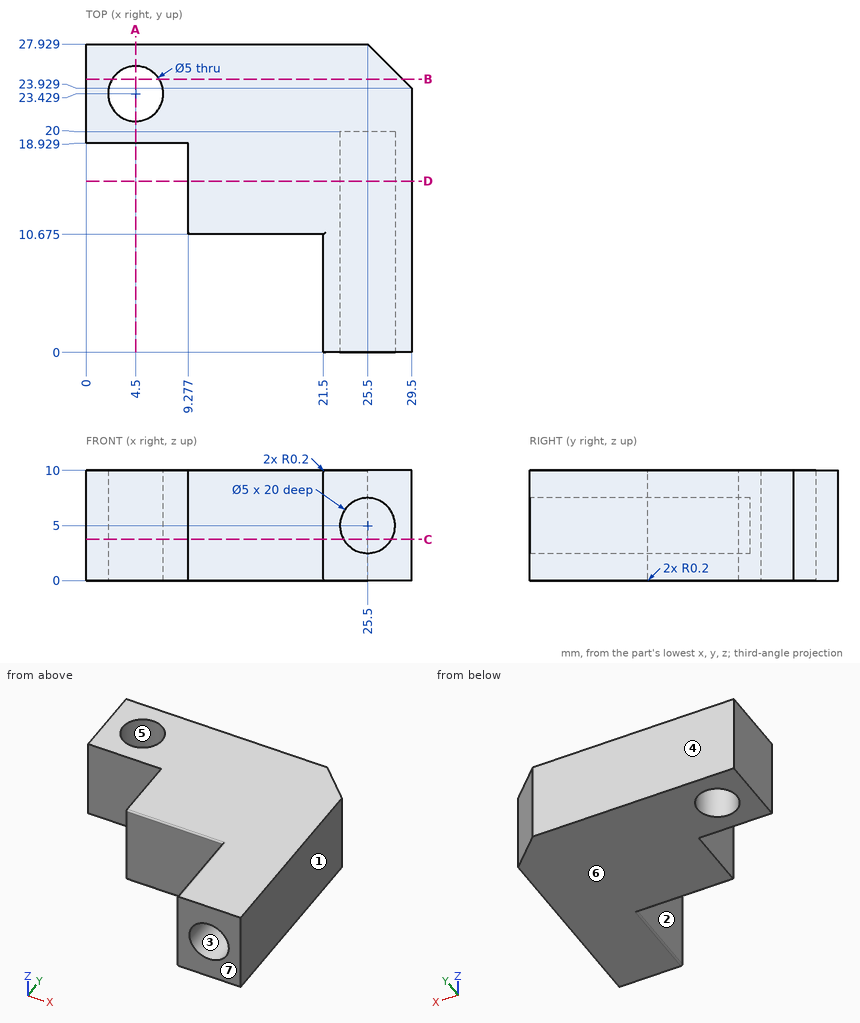
Can you work these out from the drawing? Everything is in mm from the part's minimum corner. A direction names the side the tool comes from. Give positions to 0.01 mm unless a question says otherwise; leave off trailing zeros. Order: outer loops, then holes, each group sorted by start corner. A loop starts at its lowest first (then second) coordinate and runs counter-clockwise, first axis right, second up. Notation, with made-up numbers: M 86.25,20 L 145.25,20 A8 cw 145.25,34 Z; hole C 71.5,11.25 d11. An arc over 180 degrees is marked long. Write item = value, one per line. Start each with the question number.
Q1. Suppose I cut it at C-C (z = 3.75). Write out the boundary of the cut face in (x, y) (1 decimal).
Q2. I need wall thicknesses on probe 1 along Y at (x, z) = (4.5, 3.75); probe 2 along X at (y, z) = (13, 5); probe 3 along X at (y, z) = (2, 5). Which ranges of each line are inside material? Lowest first, please. Write a range as [from, to].
Q3. Suppose I cut it at B-B (y = 24.75). Write out the boundary of the cut face in (x, z), plus the area to 3 significant figures.
Q4. Will these pins go through, and if not, where does the flat tip stop? pin 1 Ø3 at (x, z) = (3.5, 3) entering from -Y; pin 2 Ø4 at (y, z) = (13, 1) entering from -X.
Q5. Suppose I cut it at A-A (x = 4.5). Write out the boundary of the cut face in (y, z), plus the area to 3 significant figures.
Q6. For the marked faces 1, 2 and 3, which set-ups out of +Z, -Z, +X, -X, +Y, -Y let a thin tool reach every point of the face, with its end or its side?
Q7. We'd pull the mould along Y, two halves only. Please class the marked faces 4, 5, 6 and 7: pulls with the +Y half, pulls with the -Y half, needs draft (parallel to the pull), parting line crosses it, or undercut.
Q8. Suppose I cut it at D-D (y = 15.5). Write out the boundary of the cut face in (x, z), plus the area to 3 significant figures.
Check result:
q1.outline = M 0,18.9 L 9.3,18.9 L 9.3,10.7 L 21.5,10.7 L 21.5,0 L 23.3,0 L 23.3,20 L 27.7,20 L 27.7,0 L 29.5,0 L 29.5,23.9 L 25.5,27.9 L 0,27.9 Z; hole C 4.5,23.4 d5
q2.probe_1 = [18.93, 20.93], [25.93, 27.93]
q2.probe_2 = [9.28, 23], [28, 29.5]
q2.probe_3 = [21.5, 23], [28, 29.5]
q3.outline = M 0,0 L 2.38,0 L 2.38,10 L 0,10 Z; M 6.62,0 L 28.68,0 L 28.68,10 L 6.62,10 Z
q3.area = 244 mm2
q4.pin_1 = 18.93
q4.pin_2 = 9.28
q5.outline = M 18.93,0 L 20.93,0 L 20.93,10 L 18.93,10 Z; M 25.93,0 L 27.93,0 L 27.93,10 L 25.93,10 Z
q5.area = 40.0 mm2
q6.face_1 = +Z, -Z, +X, +Y, -Y
q6.face_2 = +Z, -Z, -X, -Y
q6.face_3 = -Y
q7.face_4 = pulls with the +Y half
q7.face_5 = undercut
q7.face_6 = needs draft
q7.face_7 = pulls with the -Y half
q8.outline = M 9.28,0 L 29.5,0 L 29.5,10 L 9.28,10 Z; hole C 25.5,5 d5
q8.area = 183 mm2
